from build123d import *

# Parameters (mm, degrees)
F0_W     = 151.5346497297
F0_H     = 70
F1_DEPTH = 10
F2_R     = 10
F3_R     = 5
F4_R     = 5


with BuildPart() as f1:
    # F0 (on Front) → F1 (new body, symmetric)
    with BuildSketch(Plane.XZ):
        Polygon((-300, 48), (-300, 35), (-285, 35), align=None)
        Polygon((-285, 35), (-300, 35), (-300, -35), (-285, -35), (-36.2545801078, -35), (0, -35), (0, 35), (-36.2545801078, 35), align=None)
        Polygon((-285, -35), (-300, -35), (-300, -48), align=None)
        with BuildLine():
            add(Edge.make_bspline(
                [(0, 50), (-13.1023780133, 50), (-19.1101505149, 35), (-36.2545801078, 35)],
                knots=[0, 0, 0, 0, 39.2351192019, 39.2351192019, 39.2351192019, 39.2351192019], degree=3))
            Line((-36.2545801078, 35), (0, 35))
            Line((0, 35), (0, 50))
        make_face()
        Polygon((0, 50), (0, 35), (151.5346497297, 35), (151.5346497297, -35), (0, -35), (0, -50), (253, -50), (253, 50), align=None)
        with BuildLine():
            Line((0, -35), (-36.2545801078, -35))
            add(Edge.make_bspline(
                [(-36.2545801078, -35), (-19.1101505149, -35), (-13.1023780133, -50), (0, -50)],
                knots=[0, 0, 0, 0, 39.2351192019, 39.2351192019, 39.2351192019, 39.2351192019], degree=3))
            Line((0, -50), (0, -35))
        make_face()
        with Locations((75.7673248649, 0)):
            Rectangle(F0_W, F0_H)
    extrude(amount=F1_DEPTH, both=True)

    # F2
    f2_edges = [f1.edges().sort_by_distance(p)[0] for p in [
        (253, 0, 50),
        (253, 0, -50),
    ]]
    fillet(f2_edges, radius=F2_R)

    # F3
    f3_edges = [f1.edges().sort_by_distance(p)[0] for p in [
        (-285, 0, 35),
    ]]
    fillet(f3_edges, radius=F3_R)

    # F4
    f4_edges = [f1.edges().sort_by_distance(p)[0] for p in [
        (-285, 0, -35),
    ]]
    fillet(f4_edges, radius=F4_R)


solid = f1.part
The listing builds one solid part. Answer for the finished solid, in the listing's coordinates (mm). A direction names the side the tool comes from. Give positions to 0.01 mm unless a question says otherwise; leave off trailing zeros. Write each loop counter-clockwise with the first axis right and the second up, starting at its lowest first coordinate (ties: lowest second). Pieces come first, ordered by that corner, then holes. Notation, with made-up numbers: (-3, 16.5) -> (10, 16.5) arc R26 ccw to (10, 31.5) -> close; hole circle Ø3 at (74, 10.5). An arc over 180 degrees is marked (long way). Use a Markdown table: item, result.
(1) Section A-A, the plane x = -262 is taken. Determine the outline of the cut face in (y, z).
Return value:
| item | result |
|---|---|
| outline | (-10, -35) -> (10, -35) -> (10, 35) -> (-10, 35) -> close |
(2) Find the intervals of material crossed by probe 1 along Z at (x, y) = (-175, -5); probe 2 along X at (y, z) = (5.25, 43.5); probe 3 along X at (y, z) = (-6.75, 41), in increasing order. Write a range as from..to.
Return value:
| item | result |
|---|---|
| probe 1 | -35..35 |
| probe 2 | -300..-294.81, -15.21..252.37 |
| probe 3 | -300..-291.92, -18.77..252.95 |
(3) Flat-ended cylindrical pins translate along their axes: P1, Ø10, axis at x = -243, y = -2, coming from the +Z side; P2, Ø10, axis at x = -195, y = 1.5, coming from the -Z side. Find the tip coordinate at first contact, or state that the pin passes through.
Return value:
| item | result |
|---|---|
| P1 | z = 35 |
| P2 | z = -35 |
(4) Determine the mould class of faces 4 (the cylindrical face through (249.99, -0.14, 47.15)), 5 (the flat face through (123, 0, 50)), 6 (the flat face through (-161, 0, -35)), 7 (the flat face through (-158, 0, 35)) for opening direction X: released by +X, released by -X, zero draft, split by the parting line, or undercut.
Return value:
| item | result |
|---|---|
| face 4 | released by +X |
| face 5 | zero draft |
| face 6 | undercut |
| face 7 | undercut |
(5) For faces 1 (the flat face through (-293.3, -0.14, -42.193)), 2 (the flat face through (-293.11, -0.14, 42.03)), 3 (the flat face through (-27, 10, 1)), determine the directions among +Z, -Z, +X, -X, +Y, -Y from which every point of the face is accessible in a straight line to the end or side of a thin tool.
Return value:
| item | result |
|---|---|
| face 1 | -Z, +Y, -Y |
| face 2 | +Z, +Y, -Y |
| face 3 | +Z, -Z, +X, -X, +Y |
